Could you check a few things on this model? Use its own coordinates, in mm. A direction names the side the tool comes from. Give positions to 0.01 mm unless a question says otherwise; leave off trailing zeros. Order: outer loops, then holes, each group sorted by start corner. A loop starts at its lowest first (then second) coordinate and runs counter-clockwise, first axis right, second up. Notation, with made-up numbers: (-14.5, 76) - (21.5, 76) arc R16 ccw to (21.5, 81) - close; hole circle Ø1 at (22, 4.5). An arc over 180 degrees is marked (long way). One line per question, with ' | ' between items. Start each with the question number.
1. Imagine slicing it at B-B (y = 38). Please give me the cut outline in (x, z).
2. I need wall thicknesses on probe 1 along Y at (x, z) = (-34, 118); probe 2 along Z at (x, y) = (67.5, 26.5); probe 3 along Y at (x, z) = (8.5, 104.5). Which ranges of each line are inside material? Lowest first, please. Write a range as from..to.
3. Imagine slicing it at A-A (z = 121.5). Please give me the cut outline in (x, y), and give its area (3 significant figures).
4. If we mould it in two halves opening along X, with no side actions, what happens to faces 4 (the flat face through (79, 10, 203)), 5 (the flat face through (41.1, 3.5, 190)), 6 (the flat face through (5.6, 13, 190)), 7 (the flat face through (74.204, 5, 197))? For each: released by +X, released by -X, zero draft, split by the parting line, or undercut.
5. For P1, Ø6, axis at x = 12.5, y = 30, coming from the -Z side; P2, Ø5, axis at x = -45, y = 39.5, coming from the -Z side; P3, Ø5, axis at x = 40.98, y = 6.78, coming from the -Z side (3 decimals); P4, Ø3, axis at x = 70, y = 21, coming from the +Z side, each with a flat end and sliding along its axis, tell me the tip position at first contact or that it passes through.
6. Imagine slicing it at C-C (x = -61.5). Please give me the cut outline in (y, z), and give its area (3 significant figures).
7. Which directions (+Z, -Z, +X, -X, +Y, -Y) give clear straight access to the entire face, cutting with the end or side of a thin tool? Please do faces 1 (the flat face through (79, 5, 195)), 2 (the flat face through (78, 5, 200)), 3 (the cylindrical face through (64.79, 21.02, 197.6)).
```python
from build123d import *

# Parameters (mm, degrees)
ESQUISSE1_R             = 3
BOSS_EXTRU_1_DEPTH      = 200
ESQUISSE4_W             = 5
ESQUISSE4_H             = 50
BOSS_EXTRU_4_DEPTH      = 180
BOSS_EXTRU_7_DEPTH      = 50
ESQUISSE6_W             = 20
ESQUISSE6_H             = 10.719834163
ENL_V_MAT_EXTRU_2_DEPTH = 10
ESQUISSE5_W             = 10
ESQUISSE5_H             = 10
ENL_V_MAT_EXTRU_1_DEPTH = 10
ESQUISSE14_R            = 5
ENL_V_MAT_EXTRU_4_DEPTH = 15
BOSS_EXTRU_8_REACH      = 242.401
ESQUISSE16_W            = 210.874992539
ESQUISSE16_H            = 82.741703247
ENL_V_MAT_EXTRU_5_DEPTH = 130


with BuildPart() as part:
    # Esquisse1 → Boss.-Extru.1 (new body)
    with BuildSketch(Plane.XY):
        Polygon((-105.796013405, 0), (84.203986595, 0), (84.203986595, 33.502126335), (-105.796013405, 2), align=None)
        with Locations((69.406004871, 22.939397164)):
            Circle(ESQUISSE1_R, mode=Mode.SUBTRACT)
        with Locations((40.981469067, 6.77616521)):
            Circle(ESQUISSE1_R, mode=Mode.SUBTRACT)
        with Locations((-40.796013405, 6)):
            Circle(ESQUISSE1_R, mode=Mode.SUBTRACT)
        with Locations((8.861542866, 12.901085106)):
            Circle(ESQUISSE1_R, mode=Mode.SUBTRACT)
    extrude(amount=BOSS_EXTRU_1_DEPTH)

    # Esquisse4 → Boss.-Extru.4 (add)
    with BuildSketch(Plane(origin=(84.203986595, 0, 0), x_dir=(0, 0, -1), z_dir=(1, 0, 0))):
        with Locations((-202.5, 25)):
            Rectangle(ESQUISSE4_W, ESQUISSE4_H)
        with Locations((2.5, 25)):
            Rectangle(ESQUISSE4_W, ESQUISSE4_H)
    extrude(amount=-BOSS_EXTRU_4_DEPTH)

    # Esquisse8 → Boss.-Extru.7 (add)
    with BuildSketch(Plane(origin=(0, 50, 0), x_dir=(1, 0, 0), z_dir=(0, 1, 0))):
        Polygon((84.203986595, 0), (-95.796013405, 0), (-95.796013405, -5), align=None)
    boss_extru_7 = extrude(amount=-BOSS_EXTRU_7_DEPTH)

    # Esquisse6 → Enlèv. mat.-Extru.2 (cut)
    with BuildSketch(Plane(origin=(0, 0, -5), x_dir=(-1, 0, 0), z_dir=(0, 0, -1))):
        with Locations((95.796013405, 5.359917081)):
            Rectangle(ESQUISSE6_W, ESQUISSE6_H)
    enl_v_mat_extru_2 = extrude(amount=-ENL_V_MAT_EXTRU_2_DEPTH, mode=Mode.SUBTRACT)

    # Esquisse5 → Enlèv. mat.-Extru.1 (cut)
    with BuildSketch(Plane(origin=(84.203986595, 0, 0), x_dir=(0, 0, -1), z_dir=(1, 0, 0))):
        with Locations((-200, 5)):
            Rectangle(ESQUISSE5_W, ESQUISSE5_H)
        with Locations((0, 5)):
            Rectangle(ESQUISSE5_W, ESQUISSE5_H)
    extrude(amount=-ENL_V_MAT_EXTRU_1_DEPTH, mode=Mode.SUBTRACT)

    # Esquisse14 → Enlèv. mat.-Extru.4 (cut)
    with BuildSketch(Plane(origin=(0, 0, -5), x_dir=(-1, 0, 0), z_dir=(0, 0, -1))):
        with Locations((-69.406004871, 22.939397164)):
            Circle(ESQUISSE14_R)
        with Locations((-40.981469067, 6.77616521)):
            Circle(ESQUISSE14_R)
        with Locations((-8.861542866, 12.901085106)):
            Circle(ESQUISSE14_R)
        with Locations((40.796013405, 6)):
            Circle(ESQUISSE14_R)
    enl_v_mat_extru_4 = extrude(amount=-ENL_V_MAT_EXTRU_4_DEPTH, mode=Mode.SUBTRACT)

    # Symétrie3: Boss.-Extru.7, Enlèv. mat.-Extru.2, Enlèv. mat.-Extru.4 across plane
    add(boss_extru_7.mirror(Plane(origin=(0, 0, 100), x_dir=(1, 0, 0), z_dir=(0, 0, -1))))
    add(enl_v_mat_extru_2.mirror(Plane(origin=(0, 0, 100), x_dir=(1, 0, 0), z_dir=(0, 0, -1))), mode=Mode.SUBTRACT)
    add(enl_v_mat_extru_4.mirror(Plane(origin=(0, 0, 100), x_dir=(1, 0, 0), z_dir=(0, 0, -1))), mode=Mode.SUBTRACT)

    # Boss.-Extru.8: up to this plane
    boss_extru_8_end = Plane(origin=(-95.796013405, -180.069431054, 195), z_dir=(-0.0277670672403533, 0, 0.9996144206527183))
    # Esquisse15 → Boss.-Extru.8 (add, up to the surface)
    with BuildSketch(Plane(origin=(0, 0, -5), x_dir=(-1, 0, 0), z_dir=(0, 0, -1)), mode=Mode.PRIVATE) as boss_extru_8_sk1:
        Polygon((-84.203986595, 33.502126335), (-79.203986595, 32.67312301), (-79.203986595, 50), (-84.203986595, 50), align=None)
    boss_extru_8_tool1 = split(extrude(boss_extru_8_sk1.sketch, amount=-BOSS_EXTRU_8_REACH, mode=Mode.PRIVATE), bisect_by=boss_extru_8_end, keep=Keep.BOTH, mode=Mode.PRIVATE)
    add(boss_extru_8_tool1.solids().sort_by_distance((81.683563, 41.542119, -5))[0])

    # Esquisse16 → Enlèv. mat.-Extru.5 (cut)
    with BuildSketch(Plane(origin=(0, 0, 100), x_dir=(-1, 0, 0), z_dir=(0, 0, -1))):
        with Locations((5.796013405, 25.200829376)):
            Rectangle(ESQUISSE16_W, ESQUISSE16_H)
    extrude(amount=ENL_V_MAT_EXTRU_5_DEPTH, mode=Mode.SUBTRACT)


solid = part.part
```
Results found:
1) outline: (-95.8, 195) - (79.2, 199.86) - (79.2, 100) - (84.2, 100) - (84.2, 205) - (-95.8, 205) - close
2) probe 1: y = 0..13.9 | probe 2: z = 100..190 | probe 3: y = 0..9.92, 15.88..20.95
3) outline: (-105.8, 0) - (84.2, 0) - (84.2, 50) - (79.2, 50) - (79.2, 32.67) - (-105.8, 2) - close; hole circle Ø6 at (-40.8, 6); hole circle Ø6 at (8.86, 12.9); hole circle Ø6 at (40.98, 6.78); hole circle Ø6 at (69.41, 22.94) | area: 3,340 mm2
4) face 4: zero draft | face 5: undercut | face 6: undercut | face 7: released by +X
5) P1: stops at z = 197.92 | P2: stops at z = 196.34 | P3: passes through | P4: stops at z = 190
6) outline: (0, 100) - (9.34, 100) - (9.34, 195.95) - (50, 195.95) - (50, 205) - (0, 205) - close | area: 1,350 mm2
7) face 1: +X, -Y | face 2: +Z, +X, -Y | face 3: +Z
